from build123d import *

# Parameters (mm, degrees)
F1_DEPTH       = 9.5
F3_D           = 8.8
F3_CSINK_D     = 17.92
F3_CSINK_ANGLE = 90
F4_SIZE        = 3


with BuildPart() as f1:
    # F0 (on Front) → F1 (new body)
    with BuildSketch(Plane.XZ):
        Polygon((0, -100), (0, 0), (-80, 0), (-80, -75), (-20, -75), (-20, -100), align=None)
    extrude(amount=F1_DEPTH)

    # F3 (through all)
    with Locations(Plane.XZ.offset(9.5)):
        with Locations((-62, -19), (-18.5, -57)):
            CounterSinkHole(F3_D / 2, F3_CSINK_D / 2, counter_sink_angle=F3_CSINK_ANGLE)

    # F4
    f4_edges = [f1.edges().sort_by_distance(p)[0] for p in [
        (-20, -4.75, -100),
        (0, -4.75, -100),
    ]]
    chamfer(f4_edges, length=F4_SIZE)


solid = f1.part
For this review, take the finished solid that the model builds, in its own axes (mm). A direction names the side the tool comes from. Coordinates: 2 decimals unless noted, no trailing zeros. Write each loop counter-clockwise with the first axis right and the second up, starting at its lowest first coordinate (ties: lowest second). Pieces come first, ordered by that corner, then holes. Notation, with made-up numbers: (78.25, 11.25) -> (108.25, 11.25) arc R18 cw to (108.25, 39.25) -> close; hole circle Ø10 at (-32.75, 82). An arc over 180 degrees is marked (long way). Write each question's results on one line, items separated by ' | '. Start each with the question number.
1) Consider section B-B (z = -19). Write out the cut boundary in (x, y).
2) Consider section D-D (x = -34.5). Write out the cut boundary in (y, z), plus the area to 4 significant figures.
3) For faces 4 (the face through (-20, -5, -86)), 5 (the face through (-2, -5, -99)), list the 3-axis set-ups (+Z, -Z, +X, -X, +Y, -Y) from which the entire face can be reached by the end or side of a thin tool; tool diameter is ignored.
4) Consider section C-C (y = -2). Write out the cut boundary in (x, z), plus the area to 3 significant figures.
5) The part is to be moulded in two halves that separate along X. For faces 1 (the face through (-57.604, -2.435, -18.807)), 2 (the face through (-18, -5, -99)), 3 (the face through (0, -5, -49)), say which applies: +X half, -X half, draft (parallel to the pull), parting line (faces both ways), or undercut.
6) Wall thickness on L1, parallel to X at y = -2.6, z = -57; L2, parallel to X at y = -6.5, z = -15; L3, parallel to Z at x = -62, y = -2.5: over which ranges is each line inside the solid? List them lowest first. Write a range as [from, to].
7) Insertion check: pin 1 (11.5 mm diameter, centred on x = -62, z = -19, fed in from -Y); pin 2 (1.5 mm diameter, centred on x = -51.5, y = -2, fed in from -Z); pin 3 (5 mm diameter, centred on y = -6.5, z = -86.5, fed in from -X). Each pin has a flat end and moves straight along its axis. Give the tip position at first contact, or say it passes through.
8) Consider section A-A (x = -18.5). Write out the cut boundary in (y, z), plus the area to 3 significant figures.
Geometry says:
1) outline: (-80, -9.5) -> (-70.96, -9.5) -> (-66.4, -4.94) -> (-66.4, 0) -> (-80, 0) -> close; (-57.6, -4.94) -> (-53.04, -9.5) -> (0, -9.5) -> (0, 0) -> (-57.6, 0) -> close
2) outline: (-9.5, -75) -> (0, -75) -> (0, 0) -> (-9.5, 0) -> close | area: 712.5 mm^2
3) face 4: -Z, -X, +Y, -Y | face 5: -Z, +X, +Y, -Y
4) outline: (-80, -75) -> (-20, -75) -> (-20, -97) -> (-17, -100) -> (-3, -100) -> (0, -97) -> (0, 0) -> (-80, 0) -> close; hole circle Ø8.8 at (-62, -19); hole circle Ø8.8 at (-18.5, -57) | area: 6,370 mm^2
5) face 1: undercut | face 2: -X half | face 3: +X half
6) L1: [-80, -22.9], [-14.1, 0] | L2: [-80, -66.42], [-57.58, 0] | L3: [-75, -23.4], [-14.6, 0]
7) pin 1: y = -6.29 | pin 2: z = -75 | pin 3: x = -20
8) outline: (-9.5, -98.5) -> (0, -98.5) -> (0, -61.4) -> (-4.94, -61.4) -> (-9.5, -65.96) -> close; (-9.5, -48.04) -> (-4.94, -52.6) -> (0, -52.6) -> (0, 0) -> (-9.5, 0) -> close | area: 831 mm^2
